Geometry check sheet. Reference: drawing and pictorial views, mm from the part's lowest x, y, z. Coordinates: 2 decimals unless noted, no trailing zeros. Write each loop counter-clockwise with the first axis right and the second up, starting at its lowest first coordinate (ties: lowest second). Pieces come first, ordered by that corner, then holes. Notation, with made-up numbers: M 71,0 L 97,0 A27 cw 97,35 Z; hole C 84.5,52.25 d6. An arc over 180 degrees is marked long. One line per item, written item: value.
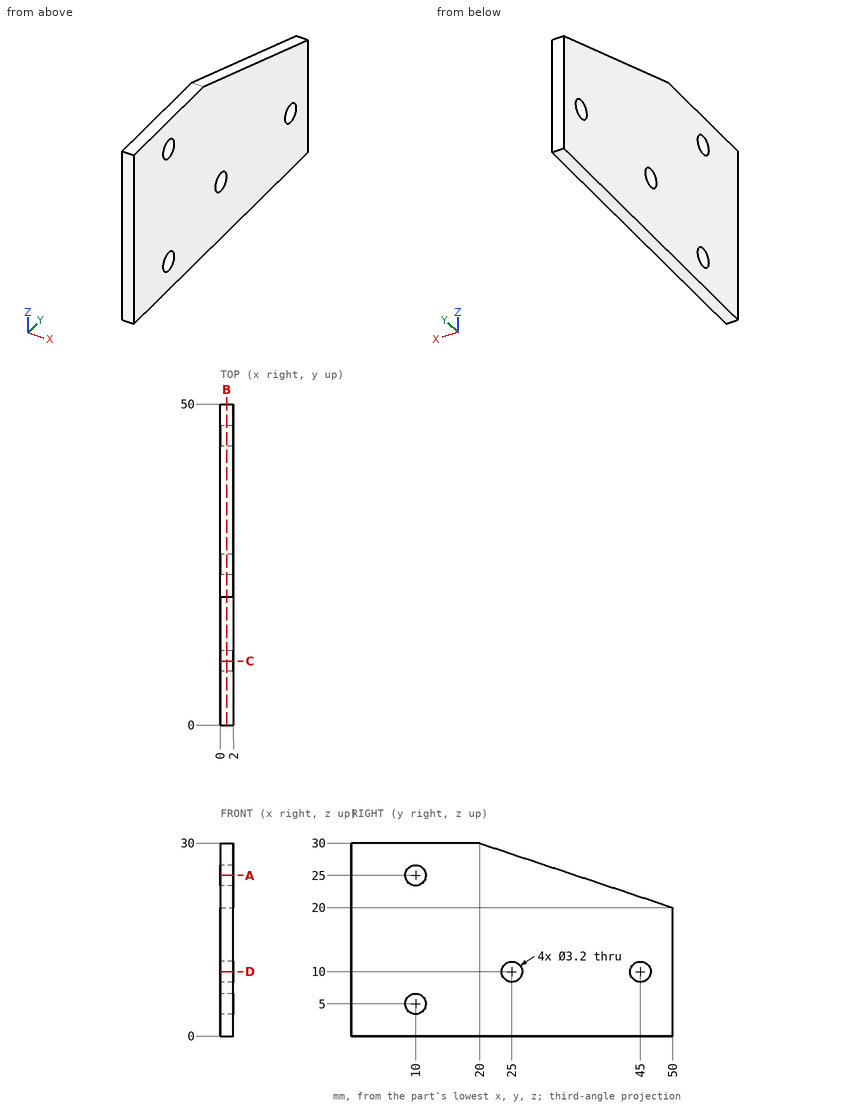
Item 1: Scan lines: line 1 (Z direction, x = 1.25, y = 10); line 2 (Y direction, x = 1.15, z = 10); line 3 (Z direction, x = 1.3, y = 9). Record each from-to range of solid material in increasing order.
The answers:
line 1: z = 0 to 3.4, 6.6 to 23.4, 26.6 to 30
line 2: y = 0 to 23.4, 26.6 to 43.4, 46.6 to 50
line 3: z = 0 to 3.75, 6.25 to 23.75, 26.25 to 30
Item 2: Cross-section at A-A, the plane z = 25. Enter the section's corners in (x, y), and give its area (3 significant figures).
The answers:
outline: M 0,0 L 2,0 L 2,8.4 L 0,8.4 Z; M 0,11.6 L 2,11.6 L 2,35 L 0,35 Z
area: 63.6 mm²
Item 3: Go/stop test with flat-tipped pins: P1, Ø1, axis at x = 1.5, y = 43.5, coming from the +Z side; P2, Ø5, axis at y = 23.5, z = 3.5, coming from the -X side; P3, Ø3, axis at y = 10, z = 25, coming from the -X side. Record where each tip stops, or that it passes through.
The answers:
P1: stops at z = 22.33
P2: stops at x = 0
P3: passes through
Item 4: Cross-section at D-D, the plane z = 10. Enter the section's corners in (x, y), and give its area (3 significant figures).
The answers:
outline: M 0,0 L 2,0 L 2,23.4 L 0,23.4 Z; M 0,26.6 L 2,26.6 L 2,43.4 L 0,43.4 Z; M 0,46.6 L 2,46.6 L 2,50 L 0,50 Z
area: 87.2 mm²
Item 5: Cross-section at C-C, the plane y = 10. Enter the section's corners in (x, z), and give its area (3 significant figures).
The answers:
outline: M 0,0 L 2,0 L 2,3.4 L 0,3.4 Z; M 0,6.6 L 2,6.6 L 2,23.4 L 0,23.4 Z; M 0,26.6 L 2,26.6 L 2,30 L 0,30 Z
area: 47.2 mm²
Item 6: Cross-section at B-B, the plane x = 0.95. Enter the section's corners in (y, z).
The answers:
outline: M 0,0 L 50,0 L 50,20 L 20,30 L 0,30 Z; hole C 10,5 d3.2; hole C 10,25 d3.2; hole C 25,10 d3.2; hole C 45,10 d3.2
